The model under review builds one solid part; all positions refer to its coordinate system, in mm. A direction names the side the tool comes from. Give positions to 0.01 mm unless a question says otherwise; leave off trailing zeros. Order: outer loops, then holes, each group sorted by start corner. A loop starts at its lowest first (then second) coordinate and runs counter-clockwise, first axis right, second up. Notation, with made-up numbers: (23.25, 35.5) - (72.25, 35.5) arc R22 ccw to (72.25, 55.5) - close; hole circle Ø1 at (22.25, 79.5). An arc over 180 degrees is marked (long way). Put each result on its own line as item: value.
```python
from build123d import *

# Parameters (mm, degrees)
SKETCH1_R           = 18
SKETCH1_R_2         = 1.75
BOSS_EXTRUDE1_DEPTH = 3
BOSS_EXTRUDE3_DEPTH = 6
CUT_EXTRUDE1_REACH  = 163.112
SKETCH4_R           = 6
CUT_EXTRUDE2_REACH  = 163.112
SKETCH5_R           = 6
CUT_EXTRUDE3_START  = -12
SKETCH1_7_R         = 1.75
CUT_EXTRUDE3_DEPTH  = 12
CUT_EXTRUDE4_START  = -12
SKETCH1_8_R         = 1.75
CUT_EXTRUDE4_DEPTH  = 12


with BuildPart() as part:
    # Sketch1 → Boss-Extrude1 (new body)
    with BuildSketch(Plane.XY):
        with BuildLine():
            Line((-45.254833996, 60.811183182), (45.254833996, 60.811183182))
            Line((45.254833996, 60.811183182), (60.811183182, 45.254833996))
            Line((60.811183182, 45.254833996), (42.526911935, 26.970562748))
            ThreePointArc((42.526911935, 26.970562748), (40.359184421, 23.72632926), (39.597979746, 19.899494937))
            Line((39.597979746, 19.899494937), (39.597979746, -19.899494937))
            ThreePointArc((39.597979746, -19.899494937), (40.359184421, -23.72632926), (42.526911935, -26.970562748))
            Line((42.526911935, -26.970562748), (60.811183182, -45.254833996))
            Line((60.811183182, -45.254833996), (45.254833996, -60.811183182))
            Line((45.254833996, -60.811183182), (-45.254833996, -60.811183182))
            Line((-45.254833996, -60.811183182), (-60.811183182, -45.254833996))
            Line((-60.811183182, -45.254833996), (-42.526911935, -26.970562748))
            ThreePointArc((-42.526911935, -26.970562748), (-40.359184421, -23.72632926), (-39.597979746, -19.899494937))
            Line((-39.597979746, -19.899494937), (-39.597979746, 19.899494937))
            ThreePointArc((-39.597979746, 19.899494937), (-40.359184421, 23.72632926), (-42.526911935, 26.970562748))
            Line((-42.526911935, 26.970562748), (-60.811183182, 45.254833996))
            Line((-60.811183182, 45.254833996), (-45.254833996, 60.811183182))
        make_face()
        Circle(SKETCH1_R, mode=Mode.SUBTRACT)
        with Locations((-37.476659403, -26.162950904)):
            Circle(SKETCH1_R_2, mode=Mode.SUBTRACT)
        with Locations((-26.162950904, -37.476659403)):
            Circle(SKETCH1_R_2, mode=Mode.SUBTRACT)
        with Locations((-40.305086528, -51.618795027)):
            Circle(SKETCH1_R_2, mode=Mode.SUBTRACT)
        with Locations((-51.618795027, -40.305086528)):
            Circle(SKETCH1_R_2, mode=Mode.SUBTRACT)
        with Locations((-22.5, 22.5)):
            Circle(SKETCH1_R_2, mode=Mode.SUBTRACT)
        with Locations((22.5, 22.5)):
            Circle(SKETCH1_R_2, mode=Mode.SUBTRACT)
        with Locations((26.162950904, 37.476659403)):
            Circle(SKETCH1_R_2, mode=Mode.SUBTRACT)
        with Locations((37.476659403, 26.162950904)):
            Circle(SKETCH1_R_2, mode=Mode.SUBTRACT)
        with Locations((51.618795027, 40.305086528)):
            Circle(SKETCH1_R_2, mode=Mode.SUBTRACT)
        with Locations((40.305086528, 51.618795027)):
            Circle(SKETCH1_R_2, mode=Mode.SUBTRACT)
        with Locations((22.5, -22.5)):
            Circle(SKETCH1_R_2, mode=Mode.SUBTRACT)
        with Locations((40.305086528, -51.618795027)):
            Circle(SKETCH1_R_2, mode=Mode.SUBTRACT)
        with Locations((51.618795027, -40.305086528)):
            Circle(SKETCH1_R_2, mode=Mode.SUBTRACT)
        with Locations((37.476659403, -26.162950904)):
            Circle(SKETCH1_R_2, mode=Mode.SUBTRACT)
        with Locations((26.162950904, -37.476659403)):
            Circle(SKETCH1_R_2, mode=Mode.SUBTRACT)
        with Locations((-22.5, -22.5)):
            Circle(SKETCH1_R_2, mode=Mode.SUBTRACT)
        with Locations((-51.618795027, 40.305086528)):
            Circle(SKETCH1_R_2, mode=Mode.SUBTRACT)
        with Locations((-40.305086528, 51.618795027)):
            Circle(SKETCH1_R_2, mode=Mode.SUBTRACT)
        with Locations((-26.162950904, 37.476659403)):
            Circle(SKETCH1_R_2, mode=Mode.SUBTRACT)
        with Locations((-37.476659403, 26.162950904)):
            Circle(SKETCH1_R_2, mode=Mode.SUBTRACT)
        with BuildLine():
            Line((-25, -55.386039841), (25, -55.386039841))
            ThreePointArc((25, -55.386039841), (30, -50.386039841), (25, -45.386039841))
            Line((25, -45.386039841), (-25, -45.386039841))
            ThreePointArc((-25, -45.386039841), (-30, -50.386039841), (-25, -55.386039841))
        make_face(mode=Mode.SUBTRACT)
        with BuildLine():
            Line((23.662950904, -10), (23.662950904, 10))
            ThreePointArc((23.662950904, 10), (26.162950904, 12.5), (28.662950904, 10))
            Line((28.662950904, 10), (28.662950904, -10))
            ThreePointArc((28.662950904, -10), (26.162950904, -12.5), (23.662950904, -10))
        make_face(mode=Mode.SUBTRACT)
        with BuildLine():
            Line((-28.662950904, -10), (-28.662950904, 10))
            ThreePointArc((-28.662950904, 10), (-26.162950904, 12.5), (-23.662950904, 10))
            Line((-23.662950904, 10), (-23.662950904, -10))
            ThreePointArc((-23.662950904, -10), (-26.162950904, -12.5), (-28.662950904, -10))
        make_face(mode=Mode.SUBTRACT)
        with BuildLine():
            Line((-25, 45.386039841), (25, 45.386039841))
            ThreePointArc((25, 45.386039841), (30, 50.386039841), (25, 55.386039841))
            Line((25, 55.386039841), (-25, 55.386039841))
            ThreePointArc((-25, 55.386039841), (-30, 50.386039841), (-25, 45.386039841))
        make_face(mode=Mode.SUBTRACT)
    extrude(amount=BOSS_EXTRUDE1_DEPTH)

    # Sketch3 → Boss-Extrude3 (add)
    with BuildSketch(Plane.XY):
        Polygon((-60.811183182, 45.254833996), (-45.254833996, 60.811183182), (-17.053249746, 32.609598932), (-32.609598932, 17.053249746), align=None)
        Polygon((-60.811183182, -45.254833996), (-32.609598932, -17.053249746), (-17.053249746, -32.609598932), (-45.254833996, -60.811183182), align=None)
        Polygon((60.811183182, -45.254833996), (45.254833996, -60.811183182), (17.053249746, -32.609598932), (32.609598932, -17.053249746), align=None)
        Polygon((60.811183182, 45.254833996), (32.609598932, 17.053249746), (17.053249746, 32.609598932), (45.254833996, 60.811183182), align=None)
    extrude(amount=-BOSS_EXTRUDE3_DEPTH)

    # Cut-Extrude1: up to this face of the body (flat: up to its plane)
    cut_extrude1_end = Plane(part.part.faces().sort_by_distance((53.033008589, -53.033008589, -1.5))[0])
    # Sketch4 → Cut-Extrude1 (cut, up to the picked face)
    with BuildSketch(Plane(origin=(-53.033008589, 53.033008589, 0), x_dir=(0, 0, 1), z_dir=(-0.7071067811865477, 0.7071067811865475, 0)), mode=Mode.PRIVATE) as cut_extrude1_sk1:
        with Locations((-8.5, 0)):
            Circle(SKETCH4_R)
    cut_extrude1_tool1 = split(extrude(cut_extrude1_sk1.sketch, amount=-CUT_EXTRUDE1_REACH, mode=Mode.PRIVATE), bisect_by=cut_extrude1_end, keep=Keep.BOTH, mode=Mode.PRIVATE)
    add(cut_extrude1_tool1.solids().sort_by(Axis((-53.033009, 53.033009, -8.5), (0.7071067811865477, -0.7071067811865475, 0)))[0], mode=Mode.SUBTRACT)

    # Cut-Extrude2: up to this face of the body (flat: up to its plane)
    cut_extrude2_end = Plane(part.part.faces().sort_by_distance((53.033008589, 53.033008589, -1.5))[0])
    # Sketch5 → Cut-Extrude2 (cut, up to the picked face)
    with BuildSketch(Plane(origin=(-53.033008589, -53.033008589, 0), x_dir=(0, 0, 1), z_dir=(-0.7071067811865477, -0.7071067811865475, 0)), mode=Mode.PRIVATE) as cut_extrude2_sk1:
        with Locations((-8.5, 0)):
            Circle(SKETCH5_R)
    cut_extrude2_tool1 = split(extrude(cut_extrude2_sk1.sketch, amount=-CUT_EXTRUDE2_REACH, mode=Mode.PRIVATE), bisect_by=cut_extrude2_end, keep=Keep.BOTH, mode=Mode.PRIVATE)
    add(cut_extrude2_tool1.solids().sort_by(Axis((-53.033009, -53.033009, -8.5), (0.7071067811865477, 0.7071067811865475, 0)))[0], mode=Mode.SUBTRACT)

    # Sketch1<7> → Cut-Extrude3 (cut)
    with BuildSketch(Plane.XY.offset(CUT_EXTRUDE3_START)):
        with Locations((-37.476659403, -26.162950904)):
            Circle(SKETCH1_7_R)
        with Locations((-26.162950904, -37.476659403)):
            Circle(SKETCH1_7_R)
        with Locations((-40.305086528, -51.618795027)):
            Circle(SKETCH1_7_R)
        with Locations((-51.618795027, -40.305086528)):
            Circle(SKETCH1_7_R)
        with Locations((26.162950904, 37.476659403)):
            Circle(SKETCH1_7_R)
        with Locations((51.618795027, 40.305086528)):
            Circle(SKETCH1_7_R)
        with Locations((40.305086528, 51.618795027)):
            Circle(SKETCH1_7_R)
        with Locations((40.305086528, -51.618795027)):
            Circle(SKETCH1_7_R)
        with Locations((51.618795027, -40.305086528)):
            Circle(SKETCH1_7_R)
        with Locations((37.476659403, -26.162950904)):
            Circle(SKETCH1_7_R)
        with Locations((26.162950904, -37.476659403)):
            Circle(SKETCH1_7_R)
        with Locations((-51.618795027, 40.305086528)):
            Circle(SKETCH1_7_R)
        with Locations((-40.305086528, 51.618795027)):
            Circle(SKETCH1_7_R)
        with Locations((-26.162950904, 37.476659403)):
            Circle(SKETCH1_7_R)
        with Locations((-37.476659403, 26.162950904)):
            Circle(SKETCH1_7_R)
    extrude(amount=CUT_EXTRUDE3_DEPTH, mode=Mode.SUBTRACT)

    # Sketch1<8> → Cut-Extrude4 (cut)
    with BuildSketch(Plane.XY.offset(CUT_EXTRUDE4_START)):
        with Locations((37.476659403, 26.162950904)):
            Circle(SKETCH1_8_R)
    extrude(amount=CUT_EXTRUDE4_DEPTH, mode=Mode.SUBTRACT)


solid = part.part
```
(1) The part is to be moulded in two halves that separate along Y. For faces 5 (the flat face through (-24.723, 24.94, -2.291)), 6 (the flat face through (-31.351, 46.908, -2.958)), 7 (the flat face through (45, 33, -6)), 8 (the flat face through (1, -60.811, 1)), say which applies: pulls with the +Y half, pulls with the -Y half, needs draft (parallel to the pull), parting line crosses it, or undercut.
The answers:
face 5: undercut
face 6: pulls with the +Y half
face 7: needs draft
face 8: pulls with the -Y half
(2) Take a section at B-B, the plane x = 0. Write out the cut boundary in (y, z), then the cut area to 3 significant figures.
The answers:
outline: (-60.81, 0) - (-55.39, 0) - (-55.39, 3) - (-60.81, 3) - close; (-45.39, 0) - (-18, 0) - (-18, 3) - (-45.39, 3) - close; (18, 0) - (45.39, 0) - (45.39, 3) - (18, 3) - close; (55.39, 0) - (60.81, 0) - (60.81, 3) - (55.39, 3) - close
area: 197 mm^2
(3) For faces 1 (the flat face through (31.351, -46.908, -2.958)), 2 (the flat face through (0, 55.386, 1)), 3 (the cylindrical face through (40.34, -23.68, 1.48)), 4 (the flat face through (-45, 32, -6)), list the 3-axis set-ups (+Z, -Z, +X, -X, +Y, -Y) from which the entire face can be reached by the end or side of a thin tool; tool diameter is ignored.
The answers:
face 1: -Z, -Y
face 2: +Z, -Z
face 3: +Z, -Z, +X
face 4: -Z, +X, -X, +Y, -Y
(4) Clearance check with flat-ended pins moving along their axes: pin 1 Ø2 at (x, y) = (-22.5, 22.5) entering from -Z; pin 2 Ø0.9 at (y, z) = (0, 1) entering from -X; pin 3 Ø2.5 at (y, z) = (0.5, 1) entering from +X; pin 4 Ø1.5 at (x, z) = (42, -4.5) entering from +Y. State where each tip first meets the part, or that it passes through.
The answers:
pin 1: through
pin 2: x = -39.6
pin 3: x = 39.6
pin 4: y = 58.31
(5) Take a section at C-C, the plane y = -22.5. Count the separate pieces of the cut face and the enclosed holes in it, then the cut area to 3 significant figures.
The answers:
separate pieces: 3
enclosed holes: 0
area: 340 mm^2
(6) Wall thickness on L1, parallel to X at y = 1, z = 0.75; L2, parallel to Y at x = 0, z = 1.8; L3, parallel to X at y = 52, z = -3.75: over which ranges is each line inside the solid? List them lowest first.
The answers:
L1: -39.6 to -28.66, -23.66 to -17.97, 17.97 to 23.66, 28.66 to 39.6
L2: -60.81 to -55.39, -45.39 to -18, 18 to 45.39, 55.39 to 60.81
L3: -46.82 to -42.01, -38.6 to -36.44, 36.44 to 38.6, 42.01 to 46.82
(7) Take a section at A-A, the plane y = 0. Write out the cut boundary in (x, z).
The answers:
outline: (-39.6, 0) - (-28.66, 0) - (-28.66, 3) - (-39.6, 3) - close; (-23.66, 0) - (-18, 0) - (-18, 3) - (-23.66, 3) - close; (18, 0) - (23.66, 0) - (23.66, 3) - (18, 3) - close; (28.66, 0) - (39.6, 0) - (39.6, 3) - (28.66, 3) - close
